Input: part model. Units: mm. Frame: model coordinates. Coordinates: 2 decimals unless noted, no trailing zeros. Write each loop counter-clockwise with the first axis right and the second up, starting at its lowest first coordinate (ties: lowest second). Pieces come first, ordered by that corner, then holes. Notation, with made-up numbers: (73, -27.75) - (104, -27.75) arc R25 cw to (104, -6.75) - close; hole circle Ø4 at (79, -37.5). An arc over 180 degrees is marked (long way). Put each result on its own line as item: value. Start each with the question number.
1. Cut plane D-D, the plane x = 6. Return loops of the section in (y, z), and give its area (3 significant figures).
2. Cut plane A-A, the plane z = 35.5. Return loops of the section in (x, y), and give its area (3 significant figures).
3. Cut plane B-B, the plane x = -79.5. Return loops of the section in (y, z).
4. Line query: line 1 (X direction, y = -7.5, z = 21); line 2 (Z direction, x = 105.5, y = -11); line 3 (Z direction, x = 6, y = -1.25). Output: solid intervals per line, ascending.
5. Cut plane C-C, the plane y = -4.25. Return loops of the section in (x, z).
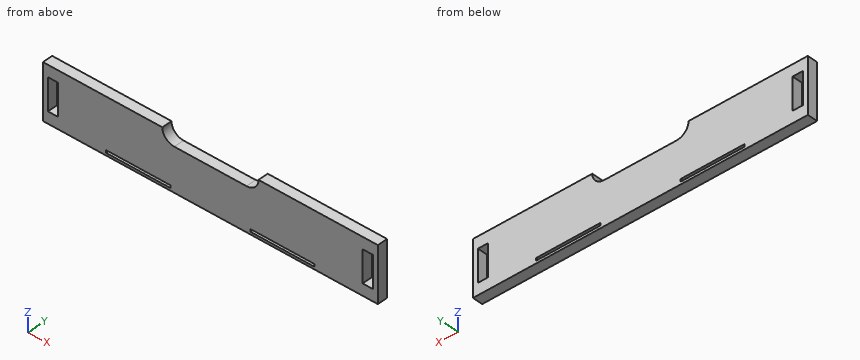
from build123d import *

# Parameters (mm, degrees)
F1_W     = 80
F1_H     = 3.18
F1_W_2   = 12.7
F1_H_2   = 40
F2_DEPTH = 12.7


with BuildPart() as f2:
    # F1 (on Front) → F2 (new body)
    with BuildSketch(Plane.XZ):
        with BuildLine():
            Line((-208.8, 65.82), (-208.8, -3.18))
            Line((-208.8, -3.18), (208.8, -3.18))
            Line((208.8, -3.18), (208.8, 65.82))
            Line((208.8, 65.82), (60, 65.82))
            ThreePointArc((60, 65.82), (55.6066017178, 55.2133982822), (45, 50.82))
            Line((45, 50.82), (-45, 50.82))
            ThreePointArc((-45, 50.82), (-55.6066017178, 55.2133982822), (-60, 65.82))
            Line((-60, 65.82), (-208.8, 65.82))
        make_face()
        with Locations((-90, 1.59)):
            Rectangle(F1_W, F1_H, mode=Mode.SUBTRACT)
        with Locations((90, 1.59)):
            Rectangle(F1_W, F1_H, mode=Mode.SUBTRACT)
        with Locations((-196.25, 31.32)):
            Rectangle(F1_W_2, F1_H_2, mode=Mode.SUBTRACT)
        with Locations((196.25, 31.32)):
            Rectangle(F1_W_2, F1_H_2, mode=Mode.SUBTRACT)
    extrude(amount=F2_DEPTH)


solid = f2.part
Report:
1. outline: (-12.7, -3.18) - (0, -3.18) - (0, 50.82) - (-12.7, 50.82) - close
1. area: 686 mm^2
2. outline: (-208.8, -12.7) - (-202.6, -12.7) - (-202.6, 0) - (-208.8, 0) - close; (-189.9, -12.7) - (189.9, -12.7) - (189.9, 0) - (-189.9, 0) - close; (202.6, -12.7) - (208.8, -12.7) - (208.8, 0) - (202.6, 0) - close
2. area: 4,980 mm^2
3. outline: (-12.7, -3.18) - (0, -3.18) - (0, 0) - (-12.7, 0) - close; (-12.7, 3.18) - (0, 3.18) - (0, 65.82) - (-12.7, 65.82) - close
4. line 1: x = -208.8 to -202.6, -189.9 to 189.9, 202.6 to 208.8
4. line 2: z = -3.18 to 0, 3.18 to 65.82
4. line 3: z = -3.18 to 50.82
5. outline: (-208.8, -3.18) - (208.8, -3.18) - (208.8, 65.82) - (60, 65.82) arc R15 cw to (45, 50.82) - (-45, 50.82) arc R15 cw to (-60, 65.82) - (-208.8, 65.82) - close; hole (-202.6, 11.32) - (-189.9, 11.32) - (-189.9, 51.32) - (-202.6, 51.32) - close; hole (-130, 0) - (-50, 0) - (-50, 3.18) - (-130, 3.18) - close; hole (50, 0) - (130, 0) - (130, 3.18) - (50, 3.18) - close; hole (189.9, 11.32) - (202.6, 11.32) - (202.6, 51.32) - (189.9, 51.32) - close
